from build123d import *

# Parameters (mm, degrees)
PAD006_DEPTH           = 32
SKETCH014_R            = 6
POCKET004_DEPTH        = 273.900652
LINEARPATTERN002_COUNT = 4
LINEARPATTERN002_PITCH = 130


with BuildPart() as part:
    # Sketch013 → Pad006 (new body)
    with BuildSketch(Plane.XY):
        Polygon((-456.887332, 341.7), (10.181459, 14.654912), (6.74, 9.74), (-460.32879, 336.785088), align=None)
    extrude(amount=PAD006_DEPTH)

    # Sketch014 (on Face3 of Pad006) → Pocket004 (cut, through all)
    with BuildSketch(Plane(origin=(6.793695, 9.702402, 0), x_dir=(0.819152, -0.573576, 0), z_dir=(-0.573576, -0.819152, 0))):
        with Locations((-462.664681, 16)):
            Circle(SKETCH014_R)
    pocket004 = extrude(amount=-POCKET004_DEPTH, mode=Mode.SUBTRACT)

    # LinearPattern002: Pocket004 ×4
    with Locations(*[Vector(0.819152, -0.573576, 0) * (i * LINEARPATTERN002_PITCH) for i in range(1, LINEARPATTERN002_COUNT)]):
        add(pocket004, mode=Mode.SUBTRACT)


with BuildPart() as part_1:
    # Body005 placement: moved
    add(part.part.moved(Location((0, 0, 9))))


solid = part_1.part
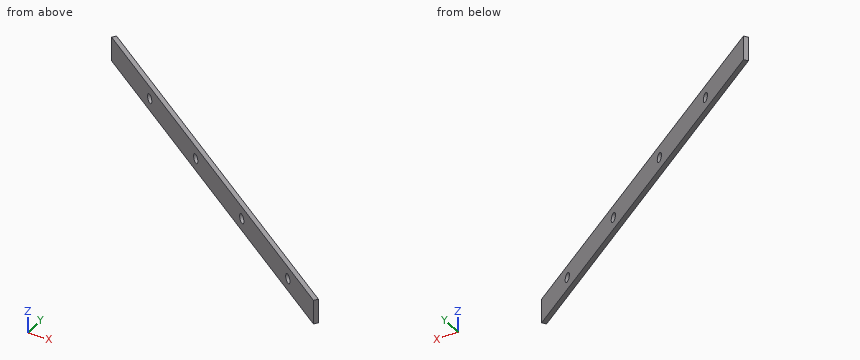
Design review of the part built by this model. Coordinates are the model's own, in mm. Coordinates: 2 decimals unless noted, no trailing zeros. Write each loop counter-clockwise with the first axis right and the second up, starting at its lowest first coordinate (ties: lowest second). Pieces come first, ordered by that corner, then holes. Notation, with made-up numbers: (43, -11.75) - (58, -11.75) arc R16 ccw to (58, 1.25) - close; hole circle Ø1 at (57.25, 81). An arc over 180 degrees is marked (long way). Use one line per item in the form item = value.
Q1. Insertion check: pin 1 Ø3 at (x, z) = (-89, 22.5) entering from -Y; pin 2 Ø6 at (y, z) = (262.5, 14.5) entering from +X; pin 3 Ø3 at (x, z) = (-293, 18) entering from -Y. Each pin has a flat end and moves straight along its axis. Give the tip position at first contact, or say it passes through.
Taken from the geometry:
pin_1 = 75.73
pin_2 = -339.49
pin_3 = 218.57
Q2. For probe 1 along X at (y, z) = (283.5, 25); probe 2 along Y at (x, z) = (-98.5, 12); probe 3 along Y at (x, z) = (-310, 33), list the stretches that pass through material, from the lowest coordinate up.
Taken from the geometry:
probe_1 = -384.23 to -373.77
probe_2 = 83.43 to 90.75
probe_3 = 231.52 to 238.85
Q3. Consider section B-B (y = 256.5). Write out the cut boundary in (x, z).
Taken from the geometry:
outline = (-345.67, 9) - (-335.21, 9) - (-335.21, 41) - (-345.67, 41) - close
Q4. Consider section A-A (x = -71.5). Write out the cut boundary in (y, z), plus the area to 3 significant figures.
Taken from the geometry:
outline = (64.52, 9) - (71.85, 9) - (71.85, 41) - (64.52, 41) - close
area = 234 mm^2
